```python
from build123d import *

# Parameters (mm, degrees)
F0_W     = 50.292
F0_H     = 85.852
F1_DEPTH = 12.7
F2_T     = -2.54
F4_DEPTH = 25.4


with BuildPart() as f1:
    # F0 (on Top) → F1 (new body)
    with BuildSketch(Plane.XY):
        with Locations((25.146, -42.926)):
            Rectangle(F0_W, F0_H)
    extrude(amount=F1_DEPTH)

    # F2
    f2_openings = [f1.faces().sort_by_distance(p)[0] for p in [
        (25.146, -42.926, 12.7),
    ]]
    offset(amount=F2_T, openings=f2_openings)

    # F3 (on face) → F4 (cut)
    with BuildSketch(Plane.XZ.offset(85.852)):
        with BuildLine():
            ThreePointArc((15.71989, 12.7), (25.146, 3.27389), (34.57211, 12.7))
            Line((34.57211, 12.7), (15.71989, 12.7))
        make_face()
    extrude(amount=-F4_DEPTH, mode=Mode.SUBTRACT)


solid = f1.part
```
Here's how the part is built. I have some questions about the finished solid (model axes, mm). A direction names the side the tool comes from. Round coordinates to 2 decimals unless told otherwise and drop trailing zeros. Loops run counter-clockwise (first coordinate to the right, second up) from the corner with the lowest first, then second, coordinate; pieces in that order, holes last.
1. Suppose I cut it at C-C, the plane z = 11.75. Please give me the cut outline in (x, y).
Answers:
outline: (0, -85.85) - (15.77, -85.85) - (15.77, -83.31) - (2.54, -83.31) - (2.54, -2.54) - (47.75, -2.54) - (47.75, -83.31) - (34.52, -83.31) - (34.52, -85.85) - (50.29, -85.85) - (50.29, 0) - (0, 0) - close
2. For faces 1 (the face through (47.752, -43, 8)), 2 (the face through (24.939, -84.6, 3.276)), 3 (the face through (1, -40, 12.7)), which set-ups out of +Z, -Z, +X, -X, +Y, -Y let a thin tool reach every point of the face, with its end or its side?
Answers:
face 1: +Z
face 2: +Z, -Y
face 3: +Z, +X, -X, +Y, -Y
3. Suppose I cut it at B-B, the plane x = 36. Please give me the cut outline in (y, z), and give its area (3 significant figures).
Answers:
outline: (-85.85, 0) - (0, 0) - (0, 12.7) - (-2.54, 12.7) - (-2.54, 2.54) - (-83.31, 2.54) - (-83.31, 12.7) - (-85.85, 12.7) - close
area: 270 mm2
4. Thinking about a two-plate mould opening in Y: for faces 4 (the face through (25, -85.852, 2)), 5 (the face through (2.54, -43, 8)), 6 (the face through (25, -42, 2.54)), 7 (the face through (0, -44, 6)), which applies, released by +Y, released by -Y, zero draft, split by the parting line, or undercut?
Answers:
face 4: released by -Y
face 5: undercut
face 6: undercut
face 7: zero draft
5. Suppose I cut it at A-A, the plane y = -19. Please give me the cut outline in (x, z), and give its area (3 significant figures).
Answers:
outline: (0, 0) - (50.29, 0) - (50.29, 12.7) - (47.75, 12.7) - (47.75, 2.54) - (2.54, 2.54) - (2.54, 12.7) - (0, 12.7) - close
area: 179 mm2
6. Will these pins go through, and if not, where does the flat tip stop? pin 1 (5 mm diameter, centred on x = 20.5, z = 11.5, fed in from -Y); pin 2 (5 mm diameter, centred on y = -35.5, z = 5, fed in from -X).
Answers:
pin 1: stops at y = -2.54
pin 2: stops at x = 0
7. If I drill on probe 1 along Y at (x, z) = (16.5, 3.25); probe 2 along X at (y, z) = (-15, 3); probe 3 along Z at (x, y) = (37.5, -3), over which ranges is the centre line in solid material (lowest first)?
Answers:
probe 1: y = -85.85 to -83.31, -2.54 to 0
probe 2: x = 0 to 2.54, 47.75 to 50.29
probe 3: z = 0 to 2.54
